Read the model definition and answer for the solid it produces. Units are mm, in the model's axes. A direction names the side the tool comes from. Coordinates: 2 decimals unless noted, no trailing zeros. Order: outer loops, then holes, each group sorted by start corner. A loop starts at its lowest first (then second) coordinate and runs counter-clockwise, first axis right, second up. Notation, with made-up numbers: M -22.5,-19 L 36.5,-19 A19 ccw 36.5,-1 Z; hole C 51,3.5 d2. An arc over 180 degrees is marked long. Use a Markdown table: item, result. Add a question column.
1) Find section C-C on y = 20. Write down the section's boundary in (x, z), plus the area to 3 significant figures.
2) Find the intervals of material crossed by probe 1 along Y at (x, z) = (-28, 4.25); probe 2 along X at (y, z) = (-50, 2.75); probe 3 along X at (y, z) = (20, 4.25), in increasing order. Write a range as [from, to].
3) Each of these flat-tipped pins is pushed along its axis until it touches: pin 1 Ø8.5 at (y, z) = (-50, 5) entering from +X; pin 2 Ø11.5 at (y, z) = (-50.5, 7.5) entering from -X; pin 3 Ø1.5 at (x, z) = (-39, 10.5) entering from -Y. Where does it stop, or does it pass through?
4) Find section B-B on x = -20. Write down the section's boundary in (y, z).
5) Find section D-D on y = -50. Write down the section's boundary in (x, z), plus the area to 3 significant figures.
6) The mould has two halves that part along Y. Classify faces 4 (the face through (-28, 20, 10)), 5 (the face through (15.189, 34, 7)), 6 (the face through (-1, -55, 17)): released by +Y, released by -Y, zero draft, split by the parting line, or undercut.
7) For faces 1 (the face through (-24, -44.568, 7)), 2 (the face through (-15.789, -50, 7)), 3 (the face through (28, 20, 10)), determine the directions among +Z, -Z, +X, -X, +Y, -Y from which every point of the face is accessible in a straight line to the end or side of a thin tool.
8) Find section A-A on z = 4.5. Write down the section's boundary in (x, y), plus the area to 3 significant figures.
from build123d import *

# Parameters (mm, degrees)
F0_W     = 110
F0_H     = 110
F1_DEPTH = 20
F2_R     = 2.5
F3_DEPTH = 10
F4_W     = 30.978008
F4_H     = 10.43164
F5_DEPTH = 15


with BuildPart() as f1:
    # F0 (on Top) → F1 (new body)
    with BuildSketch(Plane.XY):
        Rectangle(F0_W, F0_H)
    extrude(amount=F1_DEPTH)

    # F2 (on face) → F3 (cut)
    with BuildSketch(Plane(origin=(0, 0, 0), x_dir=(1, 0, 0), z_dir=(0, 0, -1))):
        with Locations((20, 50)):
            Circle(F2_R)
        with Locations((-20, 50)):
            Circle(F2_R)
        with Locations((28, -20)):
            Circle(F2_R)
        with Locations((-28, -20)):
            Circle(F2_R)
    extrude(amount=-F3_DEPTH, mode=Mode.SUBTRACT)

    # F4 (on face) → F5 (cut)
    with BuildSketch(Plane(origin=(0, 0, 0), x_dir=(1, 0, 0), z_dir=(0, 0, -1))):
        Polygon((15.189216, -11.991489), (55, -11.991489), (55, 44.56836), (55, 55), (32.581832, 55), (32.581832, 44.56836), (15.189216, 44.56836), (-15.788792, 44.56836), (-32.204367, 44.56836), (-32.204367, 55), (-55, 55), (-55, 44.56836), (-55, -11.991489), (-15.788792, -11.991489), (-15.788792, -55), (15.189216, -55), align=None)
        with Locations((-0.299788, 49.78418)):
            Rectangle(F4_W, F4_H)
    extrude(amount=-F5_DEPTH, mode=Mode.SUBTRACT)


solid = f1.part
Check result:
| question | item | result |
|---|---|---|
| 1 | outline | M -55,0 L -30.5,0 L -30.5,10 L -25.5,10 L -25.5,0 L -15.79,0 L -15.79,15 L 15.19,15 L 15.19,0 L 25.5,0 L 25.5,10 L 30.5,10 L 30.5,0 L 55,0 L 55,20 L -55,20 Z |
| 1 | area | 1,640 mm2 |
| 2 | probe 1 | y = [-55, -44.57], [11.99, 17.5], [22.5, 55] |
| 2 | probe 2 | x = [-32.2, -22.5], [-17.5, -15.79], [15.19, 17.5], [22.5, 32.58] |
| 2 | probe 3 | x = [-55, -30.5], [-25.5, -15.79], [15.19, 25.5], [30.5, 55] |
| 3 | pin 1 | stops at x = 32.58 |
| 3 | pin 2 | stops at x = -32.2 |
| 3 | pin 3 | stops at y = 11.99 |
| 4 | outline | M -55,0 L -52.5,0 L -52.5,10 L -47.5,10 L -47.5,0 L -44.57,0 L -44.57,15 L 11.99,15 L 11.99,0 L 55,0 L 55,20 L -55,20 Z |
| 5 | outline | M -55,15 L -32.2,15 L -32.2,0 L -22.5,0 L -22.5,10 L -17.5,10 L -17.5,0 L -15.79,0 L -15.79,15 L 15.19,15 L 15.19,0 L 17.5,0 L 17.5,10 L 22.5,10 L 22.5,0 L 32.58,0 L 32.58,15 L 55,15 L 55,20 L -55,20 Z |
| 5 | area | 957 mm2 |
| 6 | face 4 | undercut |
| 6 | face 5 | zero draft |
| 6 | face 6 | released by -Y |
| 7 | face 1 | -Z, +X, -X |
| 7 | face 2 | -Z, +Y, -Y |
| 7 | face 3 | -Z |
| 8 | outline | M -55,11.99 L -15.79,11.99 L -15.79,55 L -55,55 Z; M -32.2,-55 L -15.79,-55 L -15.79,-44.57 L -32.2,-44.57 Z; M 15.19,-55 L 32.58,-55 L 32.58,-44.57 L 15.19,-44.57 Z; M 15.19,11.99 L 55,11.99 L 55,55 L 15.19,55 Z; hole C -28,20 d5; hole C -20,-50 d5; hole C 20,-50 d5; hole C 28,20 d5 |
| 8 | area | 3,670 mm2 |
